Input: dimensioned drawing with shaded views. Units: mm. Origin: part minimum x, y, z. A direction names the side the tool comes from. Round coordinates to 2 decimals unless told otherwise and drop trailing zeros. Order: outer loops, then holes, each group sorted by start corner. A loop starts at its lowest first (then second) coordinate and runs counter-clockwise, first axis right, second up. Notation, with made-up numbers: M -35,63 L 13,63 A13 ccw 13,81 Z; hole C 67,76 d11. An arc over 180 degrees is marked long. Put each result on its own line as item: value. Start each with the question number.
1) Section B-B, the plane x = 56. Return loops of the section in (y, z), then the cut area to 3 significant figures.
2) Draft query along X for the marked faces 1, 2, 3 and 4. Return one class per face: pulls with the +X half, pulls with the -X half, needs draft (parallel to the pull), parting line crosses it, or undercut.
3) First-contact query: P1, Ø1.8, axis at y = 32.5, z = 3, coming from the -X side; P2, Ø1.8, axis at y = 33.5, z = 4, coming from the +X side; P3, Ø1.2, axis at x = 6.5, z = 4, coming from the +Y side. Flat tips, straight axial feed; report the tip coordinate or a pass-through.
4) Section A-A, the plane y = 38. Return loops of the section in (x, z).
5) Material intervals for probe 1 along Y at (x, z) = (31, 4.75); probe 2 along Y at (x, z) = (6, 4.05); probe 3 along Z at (x, y) = (55, 3), sorted ascending. Write a range as [from, to].
6) Section D-D, the plane z = 1.5. Return loops of the section in (x, y), then the cut area to 3 significant figures.
7) Access query for the marked faces 5, 6, 7 and 8. Directions: +Z, -Z, +X, -X, +Y, -Y. A direction counts if a zero-diameter tool reaches every point of the face in a straight line with its end or side. Return the directions, or none.
8) Section C-C, the plane z = 10. Return loops of the section in (x, y), then the cut area to 3 significant figures.
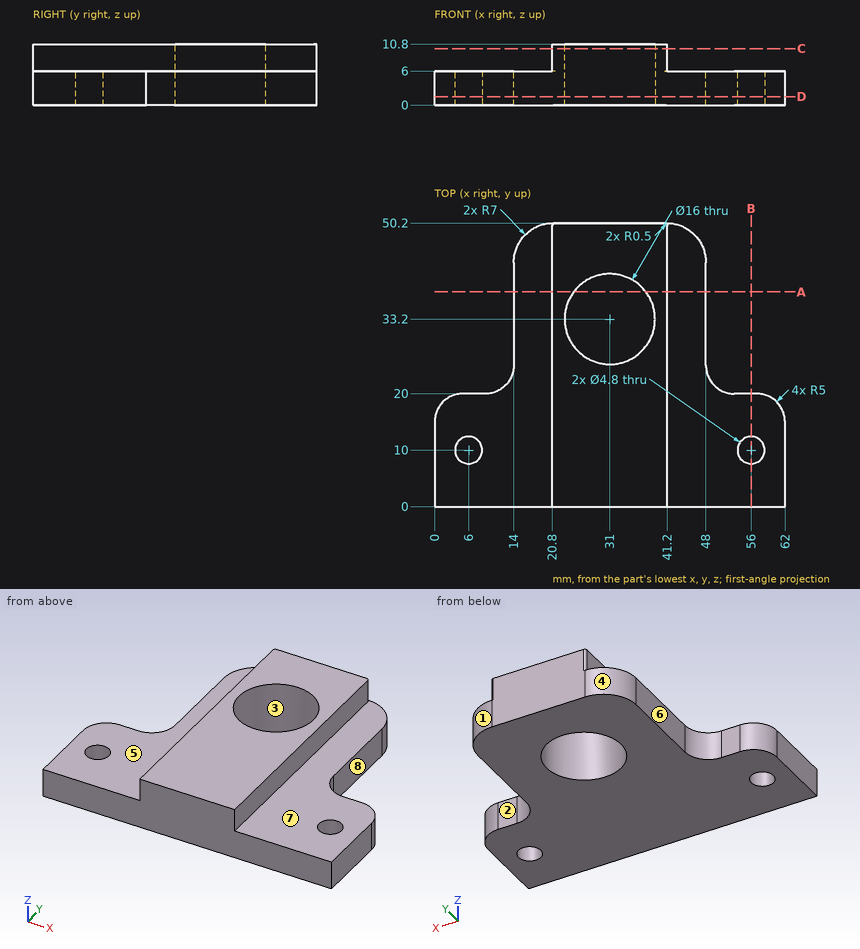
Result sheet:
1. outline: M 0,0 L 7.6,0 L 7.6,6 L 0,6 Z; M 12.4,0 L 20,0 L 20,6 L 12.4,6 Z
1. area: 91.2 mm2
2. face 1: pulls with the +X half
2. face 2: needs draft
2. face 3: undercut
2. face 4: pulls with the -X half
3. P1: stops at x = 14
3. P2: stops at x = 48
3. P3: stops at y = 20
4. outline: M 14,0 L 24.6,0 L 24.6,10.8 L 20.8,10.8 L 20.8,6 L 14,6 Z; M 37.4,0 L 48,0 L 48,6 L 41.2,6 L 41.2,10.8 L 37.4,10.8 Z
5. probe 1: y = [0, 25.2], [41.2, 50.2]
5. probe 2: y = [0, 7.6], [12.4, 20]
5. probe 3: z = [0, 6]
6. outline: M 0,0 L 62,0 L 62,15 A5 ccw 57,20 L 53,20 A5 cw 48,25 L 48,43.2 A7 ccw 41,50.2 L 21,50.2 A7 ccw 14,43.2 L 14,25 A5 cw 9,20 L 5,20 A5 ccw 0,15 Z; hole C 6,10 d4.8; hole C 31,33.2 d16; hole C 56,10 d4.8
6. area: 2,010 mm2
7. face 5: +Z, -X, +Y, -Y
7. face 6: +Z, -Z, -X, +Y
7. face 7: +Z, +X, +Y, -Y
7. face 8: +Z, -Z, +X, +Y
8. outline: M 20.8,0 L 41.2,0 L 41.2,49.7 A0.5 ccw 40.7,50.2 L 21.3,50.2 A0.5 ccw 20.8,49.7 Z; hole C 31,33.2 d16
8. area: 823 mm2
